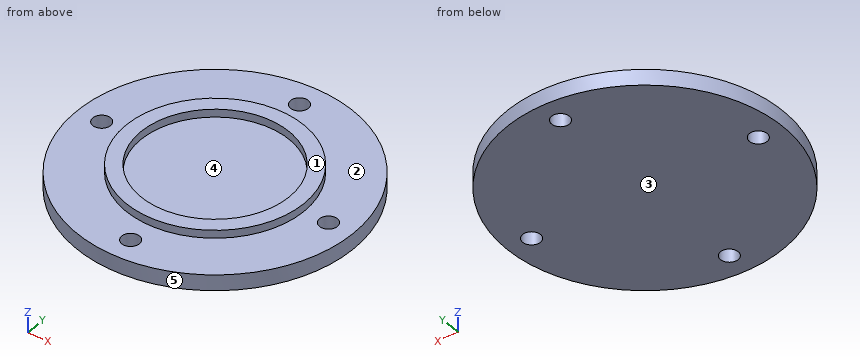
from build123d import *

# Parameters (mm, degrees)
SKETCH1_R           = 70
SKETCH1_R_2         = 4.5
BOSS_EXTRUDE1_DEPTH = 12
CUT_EXTRUDE1_START  = -4
SKETCH2_R           = 70
SKETCH2_R_2         = 45
CUT_EXTRUDE1_DEPTH  = 4
SKETCH3_R           = 37.5
CUT_EXTRUDE2_DEPTH  = 4


with BuildPart() as part:
    # Sketch1 → Boss-Extrude1 (new body)
    with BuildSketch(Plane.XY):
        Circle(SKETCH1_R)
        with Locations((0, 57.5)):
            Circle(SKETCH1_R_2, mode=Mode.SUBTRACT)
        with Locations((57.5, 0)):
            Circle(SKETCH1_R_2, mode=Mode.SUBTRACT)
        with Locations((0, -57.5)):
            Circle(SKETCH1_R_2, mode=Mode.SUBTRACT)
        with Locations((-57.5, 0)):
            Circle(SKETCH1_R_2, mode=Mode.SUBTRACT)
    extrude(amount=BOSS_EXTRUDE1_DEPTH)

    # Sketch2 → Cut-Extrude1 (cut)
    with BuildSketch(Plane.XY.offset(12).offset(CUT_EXTRUDE1_START)):
        Circle(SKETCH2_R)
        Circle(SKETCH2_R_2, mode=Mode.SUBTRACT)
    extrude(amount=CUT_EXTRUDE1_DEPTH, mode=Mode.SUBTRACT)

    # Sketch3 → Cut-Extrude2 (cut)
    with BuildSketch(Plane.XY.offset(12)):
        Circle(SKETCH3_R)
    extrude(amount=-CUT_EXTRUDE2_DEPTH, mode=Mode.SUBTRACT)


solid = part.part
The model under review builds one solid part; all positions refer to its coordinate system, in mm. Face numbers are marked on the shaded views. A direction names the side the tool comes from. Give positions to 0.01 mm unless a question says otherwise; leave off trailing zeros. Loops run counter-clockwise (first coordinate to the right, second up) from the corner with the lowest first, then second, coordinate; pieces in that order, holes last. Notation, with made-up numbers: (-32, 66) -> (12, 66) arc R23 ccw to (12, 80) -> close; hole circle Ø3 at (-29, -9). An arc over 180 degrees is marked (long way). Put each result on its own line as item: value. Start each with the question number.
1. We need section B-B on z = 5. State the section outline as (x, y) points, then the cut area to 3 significant figures.
2. We need section A-A on x = 0. State the section outline as (y, z) points, then the cut area to 3 significant figures.
3. For the marked faces 1 and 2, list the 3-axis set-ups (+Z, -Z, +X, -X, +Y, -Y) from which the entire face can be reached by the end or side of a thin tool; tool diameter is ignored.
4. We need section C-C on y = 57.5. State the section outline as (x, z) points, then the cut area to 3 significant figures.
5. Wall thickness on probe 1 along Y at (x, z) = (0, 6); probe 2 along Z at (x, y) = (33.5, 14.5); probe 3 along Y at (x, z) = (-56.5, 6.25): over which ranges is each line inside the solid? List them lowest first.
6. Mouldability with a two-part tool opening along X and no side actions: class the marked faces 3, 4 and 5 as released by +X, released by -X, zero draft, split by the parting line, or undercut.
7. Clearance check with flat-ended pins moving along their axes: P1, Ø7, axis at x = 0, y = 57.5, coming from the +Z side; P2, Ø2, axis at x = 47.5, z = 5.5, coming from the -Y side; P3, Ø1.5, axis at x = -49, z = 5, coming from the +Y side; P4, Ø3, axis at y = -33, z = 1.5, coming from the +X side. State where each tip first meets the part, or that it passes through.
Determined:
1. outline: circle Ø140 at (0, 0); hole circle Ø9 at (-57.5, 0); hole circle Ø9 at (0, -57.5); hole circle Ø9 at (0, 57.5); hole circle Ø9 at (57.5, 0)
1. area: 15,100 mm^2
2. outline: (-70, 0) -> (-62, 0) -> (-62, 8) -> (-70, 8) -> close; (-53, 0) -> (53, 0) -> (53, 8) -> (45, 8) -> (45, 12) -> (37.5, 12) -> (37.5, 8) -> (-37.5, 8) -> (-37.5, 12) -> (-45, 12) -> (-45, 8) -> (-53, 8) -> close; (62, 0) -> (70, 0) -> (70, 8) -> (62, 8) -> close
2. area: 1,040 mm^2
3. face 1: +Z, +X, -X, +Y, -Y
3. face 2: +Z
4. outline: (-39.92, 0) -> (-4.5, 0) -> (-4.5, 8) -> (-39.92, 8) -> close; (4.5, 0) -> (39.92, 0) -> (39.92, 8) -> (4.5, 8) -> close
4. area: 567 mm^2
5. probe 1: -70 to -62, -53 to 53, 62 to 70
5. probe 2: 0 to 8
5. probe 3: -41.32 to -4.39, 4.39 to 41.32
6. face 3: zero draft
6. face 4: undercut
6. face 5: split by the parting line
7. P1: through
7. P2: y = -52.32
7. P3: y = 50.71
7. P4: x = 62.51
